Read the model definition and answer for the solid it produces. Units are mm, in the model's axes. A direction names the side the tool comes from. Give positions to 0.01 mm unless a question says otherwise; leave off trailing zeros. Write each loop counter-clockwise with the first axis right and the second up, starting at its lowest first coordinate (ties: lowest second). Pieces come first, ordered by that corner, then holes. Notation, with made-up numbers: M -10,69.25 L 20,69.25 A22 cw 20,108.25 Z; hole C 12,-17 d9. An arc over 180 degrees is marked long. Write each question's results on one line, items separated by ' | '. Start each with the question number.
```python
from build123d import *

# Parameters (mm, degrees)
SKETCH1_W            = 55.892639293
SKETCH1_H            = 10
BOSS_EXTRUDE1_DEPTH  = 3
CUT_EXTRUDE1_DEPTH   = 2
M3_CLEARANCE_HOLE1_D = 3.6
BOSS_EXTRUDE2_DEPTH  = 55.892639293
BOSS_EXTRUDE3_DEPTH  = 3
M3_CLEARANCE_HOLE2_D = 3.6
CUT_EXTRUDE2_START   = -3
CUT_EXTRUDE2_DEPTH   = 2
CUT_EXTRUDE3_START   = -52.892639
CUT_EXTRUDE3_DEPTH   = 2


with BuildPart() as part:
    # Sketch1 → Boss-Extrude1 (new body)
    with BuildSketch(Plane.XY):
        with Locations((42.125546196, -5)):
            Rectangle(SKETCH1_W, SKETCH1_H)
    extrude(amount=BOSS_EXTRUDE1_DEPTH)

    # Sketch2 → Cut-Extrude1 (cut)
    with BuildSketch(Plane.XY.offset(3)):
        Polygon((65.90105946, -8.175426481), (63.15105946, -6.58771324), (63.15105946, -3.41228676), (65.90105946, -1.824573519), (68.65105946, -3.41228676), (68.65105946, -6.58771324), align=None)
        Polygon((21.100032933, -6.58771324), (21.100032933, -3.41228676), (18.350032933, -1.824573519), (15.600032933, -3.41228676), (15.600032933, -6.58771324), (18.350032933, -8.175426481), align=None)
    extrude(amount=-CUT_EXTRUDE1_DEPTH, mode=Mode.SUBTRACT)

    # M3 Clearance Hole1 (through all)
    with Locations(Plane.XY.offset(3)):
        with Locations((18.350032933, -5), (65.90105946, -5)):
            Hole(M3_CLEARANCE_HOLE1_D / 2)

    # Sketch5 → Boss-Extrude2 (add)
    with BuildSketch(Plane.ZY.offset(-14.17922655)):
        Polygon((0, 0), (21.298989873, 21.298989873), (23.420310217, 19.17766953), (3, -1.242640687), (3, 0), align=None)
    extrude(amount=-BOSS_EXTRUDE2_DEPTH)

    # Sketch6 → Boss-Extrude3 (add)
    # profile 1 of 4: a face of its own
    with BuildSketch(Plane.ZY.offset(-14.17922655)):
        with BuildLine():
            Line((11.929825022, 2.383883477), (9.278174593, 5.035533906))
            Line((9.278174593, 5.035533906), (3.373229836, -0.869410851))
            Line((3.373229836, -0.869410851), (6.024880265, -3.521061281))
            ThreePointArc((6.024880265, -3.521061281), (11.929825022, -3.521061281), (11.929825022, 2.383883477))
        make_face()
        Polygon((6.731987046, -2.8139545), (5.910126197, 0.253271947), (8.155491794, 2.498637545), (11.222718241, 1.676776695), (12.044579091, -1.390449752), (9.799213493, -3.635815349), align=None, mode=Mode.SUBTRACT)
    # profile 2 of 4: a face of its own
    with BuildSketch(Plane.ZY.offset(-14.17922655)):
        Polygon((8.155491794, 2.498637545), (11.222718241, 1.676776695), (12.044579091, -1.390449752), (9.799213493, -3.635815349), (6.731987046, -2.8139545), (5.910126197, 0.253271947), align=None)
    # profile 3 of 4: a face of its own
    with BuildSketch(Plane.ZY.offset(-14.17922655)):
        with BuildLine():
            Line((26.071960646, 16.5260191), (23.420310217, 19.17766953))
            Line((23.420310217, 19.17766953), (17.515365459, 13.272724772))
            Line((17.515365459, 13.272724772), (20.167015889, 10.621074343))
            ThreePointArc((20.167015889, 10.621074343), (26.071960646, 10.621074343), (26.071960646, 16.5260191))
        make_face()
        Polygon((23.941349117, 10.506320274), (20.87412267, 11.328181124), (20.05226182, 14.395407571), (22.297627418, 16.640773169), (25.364853865, 15.818912319), (26.186714714, 12.751685872), align=None, mode=Mode.SUBTRACT)
    # profile 4 of 4: a face of its own
    with BuildSketch(Plane.ZY.offset(-14.17922655)):
        Polygon((22.297627418, 16.640773169), (20.05226182, 14.395407571), (20.87412267, 11.328181124), (23.941349117, 10.506320274), (26.186714714, 12.751685872), (25.364853865, 15.818912319), align=None)
    boss_extrude3 = extrude(amount=-BOSS_EXTRUDE3_DEPTH)

    # Mirror1: Boss-Extrude3 across plane
    add(boss_extrude3.mirror(Plane.ZY.offset(-42.125546197)))

    # M3 Clearance Hole2 (through all)
    with Locations(Plane.ZY.offset(-14.17922655)):
        with Locations((8.977352644, -0.568588902), (23.119488267, 13.573546722)):
            Hole(M3_CLEARANCE_HOLE2_D / 2)

    # Sketch6<3> → Cut-Extrude2 (cut)
    with BuildSketch(Plane.ZY.offset(-14.17922655).offset(CUT_EXTRUDE2_START)):
        Polygon((8.155491794, 2.498637545), (11.222718241, 1.676776695), (12.044579091, -1.390449752), (9.799213493, -3.635815349), (6.731987046, -2.8139545), (5.910126197, 0.253271947), align=None)
        Polygon((22.297627418, 16.640773169), (20.05226182, 14.395407571), (20.87412267, 11.328181124), (23.941349117, 10.506320274), (26.186714714, 12.751685872), (25.364853865, 15.818912319), align=None)
    extrude(amount=CUT_EXTRUDE2_DEPTH, mode=Mode.SUBTRACT)

    # Sketch6<4> → Cut-Extrude3 (cut)
    with BuildSketch(Plane.ZY.offset(-14.17922655).offset(CUT_EXTRUDE3_START)):
        Polygon((22.297627418, 16.640773169), (20.05226182, 14.395407571), (20.87412267, 11.328181124), (23.941349117, 10.506320274), (26.186714714, 12.751685872), (25.364853865, 15.818912319), align=None)
        Polygon((8.155491794, 2.498637545), (11.222718241, 1.676776695), (12.044579091, -1.390449752), (9.799213493, -3.635815349), (6.731987046, -2.8139545), (5.910126197, 0.253271947), align=None)
    extrude(amount=-CUT_EXTRUDE3_DEPTH, mode=Mode.SUBTRACT)


solid = part.part
```
Item 1: Section D-D, the plane x = 19 is taken. Determine the outline of the cut face in (y, z).
Item 2: Determine the mould class of faces 4 (the flat face through (14.179, 8, 12)), 5 (the flat face through (42, -6, 3)), 6 (the flat face through (41.73, 9.11, 13.35)) for opening direction X: +X half, -X half, draft (parallel to the pull), parting line (faces both ways), or undercut.
Item 3: Section B-B, the plane z = 19.25 is taken. Determine the outline of the cut face in (x, y).
Item 4: Section A-A, the plane x = 53.5 is taken. Determine the outline of the cut face in (y, z), then the cut area to 3 significant figures.
Item 5: Given P1, Ø5, axis at x = 31, z = 9.5, coming from the +Y side; P2, Ø6, axis at x = 18.35, y = -5, coming from the +Z side; P3, Ø6, axis at x = 61.5, y = -4, coming from the +Z side, each flat-ended and moving along its own axis, determine where each tip first touches the part or whether it passes through.
Item 6: For faces 1 (the flat face through (68.593, -2.177, 4.68)), 2 (the flat face through (19.71, -7.39, 2.01)), 3 (the flat face through (16.19, 12.88, 20.46)), determine the directions among +Z, -Z, +X, -X, +Y, -Y from which every point of the face is accessible in a straight line to the end or side of a thin tool.
Item 7: Straight lines are drawn through the part: line 1 (X direction, y = 10.5, z = 21); line 2 (X direction, y = -2, z = 6.75); line 3 (Z direction, x = 40.5, y = -2.5). For each, find the intervals that lie inside material, in ascending order.
Item 8: Section C-C, the plane y = 4 is taken. Determine the outline of the cut face in (x, z).
Worked out:
1) outline: M -10,0 L -6.68,0 L -6.68,1 L -7.8,1 L -7.8,3 L -10,3 Z; M -3.32,0 L 0,0 L 21.3,21.3 L 19.18,23.42 L -1.24,3 L -2.2,3 L -2.2,1 L -3.32,1 Z
2) face 4: -X half | face 5: draft | face 6: undercut
3) outline: M 14.18,11.54 L 17.18,11.54 L 17.18,15.01 L 67.07,15.01 L 67.07,11.54 L 70.07,11.54 L 70.07,19.25 L 14.18,19.25 Z
4) outline: M -10,0 L 0,0 L 21.3,21.3 L 19.18,23.42 L -1.24,3 L -10,3 Z | area: 117 mm²
5) P1: stops at y = 12 | P2: stops at z = 12.8 | P3: stops at z = 3.24
6) face 1: +X, -X, -Y | face 2: +Z | face 3: none
7) line 1: x = 14.18 to 17.18, 67.07 to 70.07 | line 2: x = 14.18 to 15.18, 69.07 to 70.07 | line 3: z = 0 to 3
8) outline: M 14.18,4 L 70.07,4 L 70.07,10.31 L 67.07,10.31 L 67.07,8.24 L 17.18,8.24 L 17.18,10.31 L 14.18,10.31 Z
